For this review, take the finished solid that the model builds, in its own axes (mm). Face numbers are marked on the shaded views. A direction names the side the tool comes from. Coordinates: 2 decimals unless noted, no trailing zeros. Write each loop counter-clockwise with the first axis right and the second up, starting at its lowest first coordinate (ties: lowest second). Pieces come first, ordered by that corner, then holes. Notation, with made-up numbers: (6, 0) -> (61, 0) arc R34 cw to (61, 31) -> close; hole circle Ø9 at (-9, 76.25). An arc over 180 degrees is marked (long way). Put each result on its own line as item: value. Start each with the question number.
Item 1: For the marked faces 1 and 2, list the 3-axis set-ups (+Z, -Z, +X, -X, +Y, -Y) from which the entire face can be reached by the end or side of a thin tool; tool diameter is ignored.
Item 2: To check wall thickness, follow L1, parallel to X at y = 0.75, z = -0.5; L2, parallel to Z at x = 0.55, y = 0.8; L3, parallel to Y at x = -0.5, z = 3.25 (3 decimals). State the ranges of each line that lie inside material, in increasing order.
Item 3: Consider section C-C on z = 2. Give the boundary of the cut face in (x, y) (3 decimals), and give its area (3 significant figures).
Item 4: Consider section A-A on y = 0. Give the boundary of the cut face in (x, z) (3 decimals).
Item 5: Consider section B-B on x = 0. Give the boundary of the cut face in (y, z) (3 decimals).
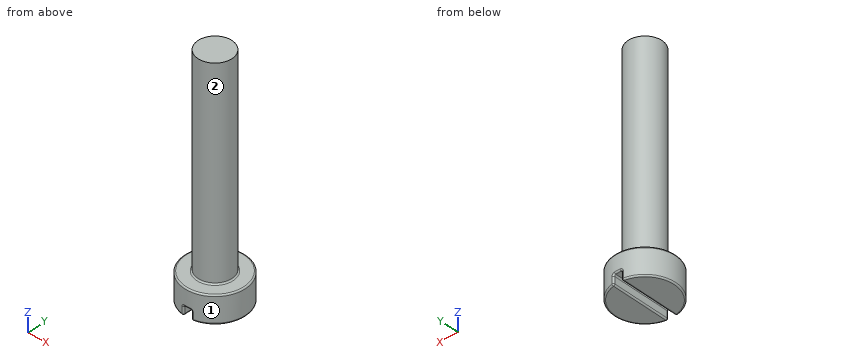
```python
from build123d import *

# Parameters (mm, degrees)
SKETCH1_R           = 0.625
BOSS_EXTRUDE1_DEPTH = 7.5
SKETCH2_R           = 1.125
BOSS_EXTRUDE2_DEPTH = 1
SKETCH3_W           = 0.3
SKETCH3_H           = 13.562630166
CUT_EXTRUDE1_DEPTH  = 0.35
FILLET1_R           = 0.05
FILLET2_R           = 0.05


with BuildPart() as part:
    # Sketch1 → Boss-Extrude1 (new body)
    with BuildSketch(Plane.XY):
        Circle(SKETCH1_R)
    extrude(amount=BOSS_EXTRUDE1_DEPTH)

    # Sketch2 → Boss-Extrude2 (add)
    with BuildSketch(Plane.XY):
        Circle(SKETCH2_R)
    extrude(amount=-BOSS_EXTRUDE2_DEPTH)

    # Sketch3 → Cut-Extrude1 (cut)
    with BuildSketch(Plane(origin=(0, 0, -1), x_dir=(-1, 0, 0), z_dir=(0, 0, -1))):
        Rectangle(SKETCH3_W, SKETCH3_H)
    extrude(amount=-CUT_EXTRUDE1_DEPTH, mode=Mode.SUBTRACT)

    # Fillet1
    fillet1_edges = [part.edges().sort_by_distance(p)[0] for p in [
        (0.846869234, -0.740565662, -1),
        (-0.15, 0, -1),
        (0.15, 0, -1),
        (0, 1.125, -0.65),
        (0, -1.125, -0.65),
        (0.15, 1.114955156, -0.825),
        (0.15, -1.114955156, -0.825),
        (-0.15, -1.114955156, -0.825),
        (-0.15, 1.114955156, -0.825),
        (0.15, 0, -0.65),
        (-0.15, 0, -0.65),
        (-1.125, 0, -1),
    ]]
    fillet(fillet1_edges, radius=FILLET1_R)

    # Fillet2
    fillet2_edges = [part.edges().sort_by_distance(p)[0] for p in [
        (-0.625, 0, 0),
        (-1.125, 0, 0),
    ]]
    fillet(fillet2_edges, radius=FILLET2_R)


solid = part.part
```
Return value:
1. face 1: +Z, -Z
1. face 2: +Z
2. L1: -0.84 to 0.84
2. L2: -1 to 0
2. L3: -0.375 to 0.375
3. outline: circle Ø1.25 at (0, 0)
3. area: 1.23 mm^2
4. outline: (-1.125, -0.95) arc R0.05 ccw to (-1.075, -1) -> (-0.2, -1) arc R0.05 ccw to (-0.15, -0.95) -> (-0.15, -0.7) arc R0.05 cw to (-0.1, -0.65) -> (0.1, -0.65) arc R0.05 cw to (0.15, -0.7) -> (0.15, -0.95) arc R0.05 ccw to (0.2, -1) -> (1.075, -1) arc R0.05 ccw to (1.125, -0.95) -> (1.125, -0.05) arc R0.05 ccw to (1.075, 0) -> (0.675, 0) arc R0.05 cw to (0.625, 0.05) -> (0.625, 7.5) -> (-0.625, 7.5) -> (-0.625, 0.05) arc R0.05 cw to (-0.675, 0) -> (-1.075, 0) arc R0.05 ccw to (-1.125, -0.05) -> close
5. outline: (-1.125, -0.6) arc R0.05 ccw to (-1.075, -0.65) -> (1.075, -0.65) arc R0.05 ccw to (1.125, -0.6) -> (1.125, -0.05) arc R0.05 ccw to (1.075, 0) -> (0.675, 0) arc R0.05 cw to (0.625, 0.05) -> (0.625, 7.5) -> (-0.625, 7.5) -> (-0.625, 0.05) arc R0.05 cw to (-0.675, 0) -> (-1.075, 0) arc R0.05 ccw to (-1.125, -0.05) -> close
